Source: CAD feature listing. Evaluate the final solid. Frame: model axes, mm. A direction names the side the tool comes from. Round coordinates to 2 decimals unless told otherwise and drop trailing zeros. Loops run counter-clockwise (first coordinate to the right, second up) from the corner with the lowest first, then second, coordinate; pieces in that order, holes last.
(1) Section C-C, the plane y = 1. Return the cut outline in (x, z) (3 decimals), plus the area to 3 significant figures.
(2) Mould query, pull axis Y, two halves, no side actions, for faces 4 (the flat face through (-2.3, 3, -0.1)), 5 (the cylindrical face through (6.232, 8.713, -1.411)), 6 (the cylindrical face through (-4.699, 1.521, 5.715)). Classes: pulls with the +Y half, pulls with the -Y half, needs draft (parallel to the pull), parting line crosses it, or undercut.
(3) Section D-D, the plane x = 6.75. Return the cut outline in (y, z) (3 decimals), plus the area to 3 significant figures.
(4) Section A-A, the plane x = 0. Return the cut outline in (y, z) (3 decimals).
(5) Material intervals for probe 1 along Y at (x, z) = (6.5, 0) (3 decimals); probe 2 along X at (y, z) = (1.3, 0) (3 decimals); probe 3 along Y at (x, z) = (-0.25, 2.75), sorted ascending.
(6) Section B-B, the plane z = 0. Return the cut outline in (x, y) (3 decimals), plus the area to 3 significant figures.
(7) First-contact query: pin 1 Ø3 at (x, z) = (-2, -1) entering from +Y; pin 2 Ø1.6 at (y, z) = (6, 0) entering from -X. Flat tips, straight axial feed; report the tip coordinate or a pass-through.
(8) Set-up query: faces 1 (the flat face through (7.5, 7, 0)), 2 (the cylindrical face through (-4.699, 1.521, -5.715)), 3 (the flat face through (5, 6, 3)). Return all of +Z, -Z, +X, -X, +Y, -Y with unobstructed straight access to the full face (end or side cutting, diameter ignored); none if empty.
```python
from build123d import *

# Parameters (mm, degrees)
SKETCH_1_W          = 13
SKETCH_1_H          = 12
EXTRUDE_1_DEPTH     = 10
SHELL_1_T           = -3
SKETCH_2_R          = 2.125
CUT_EXTRUDE_1_DEPTH = 13.206555616
SKETCH_3_R          = 2.625
CUT_EXTRUDE_4_DEPTH = 2.5
FILLET_1_R          = 1


with BuildPart() as part:
    # 草圖1 → 填料-伸長1 (new body)
    with BuildSketch(Plane(origin=(0, 0, 0), x_dir=(1, 0, 0), z_dir=(0, 1, 0))):
        with Locations((1.5, 0)):
            Rectangle(SKETCH_1_W, SKETCH_1_H)
    extrude(amount=EXTRUDE_1_DEPTH)

    # 薄殼1
    shell_1_openings = [part.faces().sort_by_distance(p)[0] for p in [
        (1.5, 10, 0),
        (1.5, 5, -6),
        (1.5, 5, 6),
        (-5, 5, 0),
    ]]
    offset(amount=SHELL_1_T, openings=shell_1_openings, kind=Kind.INTERSECTION)

    # 草圖2 → 除料-伸長1 (cut, through all)
    with BuildSketch(Plane(origin=(0, 3, 0), x_dir=(1, 0, 0), z_dir=(0, 1, 0))):
        with Locations(Location((0, 0, 0), (0, 0, 270))):
            Circle(SKETCH_2_R)
    extrude(amount=-CUT_EXTRUDE_1_DEPTH, mode=Mode.SUBTRACT)

    # 草圖3 → 除料-伸長4 (cut)
    with BuildSketch(Plane(origin=(5, 0, 0), x_dir=(0, 0, -1), z_dir=(1, 0, 0))):
        with Locations((0, 6.5)):
            Circle(SKETCH_3_R)
    extrude(amount=CUT_EXTRUDE_4_DEPTH, mode=Mode.SUBTRACT)

    # 圓角1
    fillet_1_edges = [part.edges().sort_by_distance(p)[0] for p in [
        (6.5, 10, -6),
        (-5, 1.5, -6),
        (-5, 1.5, 6),
        (6.5, 10, 6),
    ]]
    fillet(fillet_1_edges, radius=FILLET_1_R)


solid = part.part
```
Output values:
1. outline: (-5, -5) arc R1 ccw to (-4, -6) - (8, -6) - (8, 6) - (-4, 6) arc R1 ccw to (-5, 5) - close; hole circle Ø4.25 at (0, 0)
1. area: 141 mm2
2. face 4: pulls with the +Y half
2. face 5: undercut
2. face 6: needs draft
3. outline: (0, -6) - (9, -6) arc R1 ccw to (10, -5) - (10, 5) arc R1 ccw to (9, 6) - (0, 6) - close; hole circle Ø5.25 at (6.5, 0)
3. area: 97.9 mm2
4. outline: (0, -6) - (3, -6) - (3, -2.125) - (0, -2.125) - close; (0, 2.125) - (3, 2.125) - (3, 6) - (0, 6) - close
5. probe 1: y = 0 to 3.875, 9.125 to 10
5. probe 2: x = -5 to -2.125, 2.125 to 8
5. probe 3: y = 0 to 3
6. outline: (-5, 0) - (-2.125, 0) - (-2.125, 3) - (-5, 3) - close; (2.125, 0) - (8, 0) - (8, 10) - (5, 10) - (5, 9.125) - (7.5, 9.125) - (7.5, 3.875) - (5, 3.875) - (5, 3) - (2.125, 3) - close
6. area: 34.1 mm2
7. pin 1: stops at y = 3
7. pin 2: stops at x = 7.5
8. face 1: -X
8. face 2: -Z, -X, +Y, -Y
8. face 3: +Z, -Z, -X, +Y
